Autodesk Inventor part; units mm, degrees
ref_plane "YZ Plane" through (0, 0, 0) normal (1, 0, 0) x (0, 1, 0)
ref_plane "XZ Plane" through (0, 0, 0) normal (0, 1, 0) x (-1, 0, 0)
ref_plane "XY Plane" through (0, 0, 0) normal (0, 0, 1) x (1, 0, 0)
sketch "Skizze1" plane through (0, 0, 0) normal (0, 0, 1) x (1, 0, 0)
  line L0 (-7, 0) -> (7, 0)
  line L1 (0, -7) -> (0, 7)
  circle A0 centre (0, 0) radius 5
  dimension "d0" = 10
extrude "Extrusion1" add sketch "Skizze1" along normal blind 90
sketch "Skizze2" plane through (0, 0, 90) normal (0, 0, 1) x (1, 0, 0)
  point P0 (0, 0)
  point P1 (0, 0)
hole "Bohrung1" at (0, 0, 90) direction (0, 0, -1) diameter 4.134 depth 14.2 tip angle 118
sketch "Skizze3" plane through (0, 0, 0) normal (0, 0, -1) x (-1, 0, 0)
  point P0 (0, 0)
  point P1 (-2.4827, -3.6773)
hole "Bohrung2" at (0, 0, 0) direction (0, 0, 1) diameter 4.134 depth 14.2 tip angle 118
properties part number "24_0497_0020"
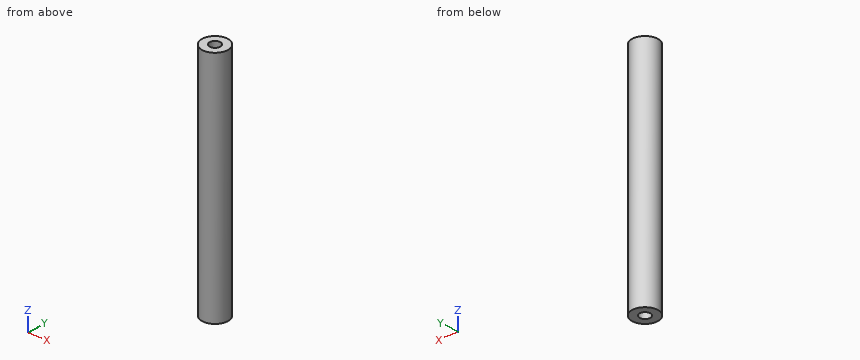
Check sheet for the modelled part. Datum: model origin and axes. Units: mm. Round coordinates to 2 decimals unless told otherwise and drop trailing zeros. Loops run counter-clockwise (first coordinate to the right, second up) from the corner with the lowest first, then second, coordinate; pieces in that order, holes last. Notation, with made-up numbers: (63.5, 26.25) -> (107.5, 26.25) arc R19 cw to (107.5, 62.25) -> close; hole circle Ø5 at (-16.5, 51.25). An arc over 180 degrees is marked (long way). Write item = value, one per line. Start each with the question number.
1) Thickness scan on probe 1 along X at (y, z) = (0, 85.75); probe 2 along Y at (x, z) = (-1, 9). Record the ranges inside material, lowest first.
2) Gauge pin test, flat ends, axial feed: pin 1 Ø2.5 at (x, y) = (0, 0) entering from -Z; pin 2 Ø4 at (y, z) = (3.5, 65) entering from +X. Record the tip position at first contact, or that the pin passes through.
3) Sectioned sample at C-C, the plane x = 3.25. Record the cut outline in (y, z).
4) Sectioned sample at B-B, the plane z = 60. Record the cut outline in (x, y).
5) Sectioned sample at A-A, the plane z = 12. Record the cut outline in (x, y).
Results are:
q1.probe_1 = -5 to -2.07, 2.07 to 5
q1.probe_2 = -4.9 to -1.81, 1.81 to 4.9
q2.pin_1 = 14.69
q2.pin_2 = 4.77
q3.outline = (-3.8, 0) -> (3.8, 0) -> (3.8, 90) -> (-3.8, 90) -> close
q4.outline = circle Ø10 at (0, 0)
q5.outline = circle Ø10 at (0, 0); hole circle Ø4.13 at (0, 0)
